Autodesk Inventor part; units mm, degrees
ref_plane "YZ Plane" through (0, 0, 0) normal (1, 0, 0) x (0, 1, 0)
ref_plane "XZ Plane" through (0, 0, 0) normal (0, 1, 0) x (-1, 0, 0)
ref_plane "XY Plane" through (0, 0, 0) normal (0, 0, 1) x (1, 0, 0)
sketch "Sketch1" plane through (0, 0, 0) normal (0, 1, 0) x (-1, 0, 0)
  line L0 (0, 0) -> (-34, 0)
  line L1 (-34, 0) -> (-34, -40)
  line L2 (-34, -40) -> (0, -40)
  line L3 (0, -40) -> (0, 0)
  dimension "d0" = 40
  dimension "d1" = 34
extrude "Extrusion1" add sketch "Sketch1" along normal blind 1.5
sketch "Sketch2" plane through (34, 0, 0) normal (1, 0, 0) x (0, 0, -1)
  line L0 (0, 1.5) -> (40, 1.5)
  line L1 (8.1604, 1.5) -> (27.7337, 21)
  line L2 (27.7337, 21) -> (22.8205, 21)
  line L3 (22.8205, 21) -> (36.5617, 1.5)
  circle A0 centre (25.2771, 21) radius 12.5
  line L4 (0, 0) -> (40, 0)
  point P0 (17.731, 11.0347)
  point P1 (30.7424, 9.7581)
  dimension "d4" = 25
  dimension "d5" = 21
extrude "Extrusion2" add sketch "Sketch2" against normal up to surface (34 mm away) contours L1 A0 L3 L0 | L3 L2 L1 | A0 L3 L1 | L1 L3 A0
sketch "Sketch3" plane through (34, 0, -40) normal (0, 0, -1) x (-1, 0, 0)
  line L0 (34, 1.5) -> (0, 1.5)
  line L1 (0, 33.5) -> (34, 33.5)
  line L2 (0, 1.5) -> (6, 1.5)
  line L3 (6, 1.5) -> (6, 33.5)
  line L4 (6, 33.5) -> (0, 33.5)
  line L5 (0, 33.5) -> (0, 1.5)
  line L6 (34, 33.5) -> (28, 33.5)
  line L7 (28, 33.5) -> (28, 1.5)
  line L8 (28, 1.5) -> (34, 1.5)
  line L9 (34, 1.5) -> (34, 33.5)
  point P0 (34, 0)
  point P1 (28, 1.5)
  dimension "d8" = 6
  dimension "d9" = 6
extrude "Extrusion3" cut sketch "Sketch3" against normal through all contours L0 L7 L1 L9 | L0 L5 L1 L3
properties part number "Rueda loca"
Part model, mm, in its own coordinate system. A direction names the side the tool comes from. Round coordinates to 2 decimals unless told otherwise and drop trailing zeros. Loops run counter-clockwise (first coordinate to the right, second up) from the corner with the lowest first, then second, coordinate; pieces in that order, holes last.
Item 1: Drop flat-ended pins along their axis: P1, Ø5, axis at x = 15.5, z = -16, coming from the +Y side; P2, Ø10, axis at x = 13, y = 10.5, coming from the -Z side; P3, Ø1, axis at y = 22.5, z = -30.5, coming from the -X side. Give the stop position or say it passes through.
Item 2: Cut at D-D, the plane z = -14. Give the cut face in (x, y).
Item 3: Cut at C-C, the plane y = 21. Give the cut face in (x, z), then the cut area to 3 significant figures.
Item 4: Cut at A-A, the plane z = -34. Give the cut face in (x, y), then the cut area to 3 significant figures.
Item 5: Mould opens along Y. For faces 1 (the face through (17.154, 33.388, -26.948)), 2 (the face through (17.2, 5.7, -33.6)), 3 (the face through (17, 0, -20)), 4 (the face through (0, 1, -20)) say: +Y half, -Y half, draft (parallel to the pull), parting line (faces both ways), or undercut.
Item 6: Cut at B-B, the plane x = 11. Give the cut face in (y, z), then the cut area to 3 significant figures.
Item 7: 3-axis set-ups, long thin cutter, end or side, ignore diameter. For faces 5 (the face through (34, 1, -20)), 6 (the face through (28, 17, -23)), 7 (the face through (6, 18, -23)), 8 (the face through (17.15, 6.2, -12.88)), 9 (the face through (17, 1, -40)): which of +Z, -Z, +X, -X, +Y, -Y reach the whole face in a straight line?
Item 8: Drill centre lines: line 1 (Y direction, x = 12, z = -6.5); line 2 (X direction, y = 7, z = -24.5); line 3 (Z direction, x = 12, y = 21). Where is each one in solid material? Low to high.
A:
1. P1: stops at y = 31.5
1. P2: stops at z = -36.5
1. P3: stops at x = 6
2. outline: (0, 0) - (34, 0) - (34, 1.5) - (28, 1.5) - (28, 7.32) - (6, 7.32) - (6, 1.5) - (0, 1.5) - close; (6, 15.61) - (28, 15.61) - (28, 26.39) - (6, 26.39) - close
3. outline: (6, -37.78) - (28, -37.78) - (28, -12.78) - (6, -12.78) - close
3. area: 550 mm2
4. outline: (0, 0) - (34, 0) - (34, 1.5) - (28, 1.5) - (28, 5.14) - (6, 5.14) - (6, 1.5) - (0, 1.5) - close; (6, 12.05) - (28, 12.05) - (28, 29.95) - (6, 29.95) - close
4. area: 525 mm2
5. face 1: undercut
5. face 2: undercut
5. face 3: -Y half
5. face 4: draft
6. outline: (0, -40) - (1.5, -40) - (1.5, -36.56) - (9.76, -30.74) arc R12.5 ccw (long way) to (11.03, -17.73) - (1.5, -8.16) - (1.5, 0) - (0, 0) - close
6. area: 720 mm2
7. face 5: +Z, -Z, +X, +Y, -Y
7. face 6: +Z, -Z, +X, +Y
7. face 7: +Z, -Z, -X, +Y
7. face 8: +Z, +X, -X
7. face 9: -Z, +X, -X, +Y, -Y
8. line 1: y = 0 to 1.5
8. line 2: x = 6 to 28
8. line 3: z = -37.78 to -12.78
